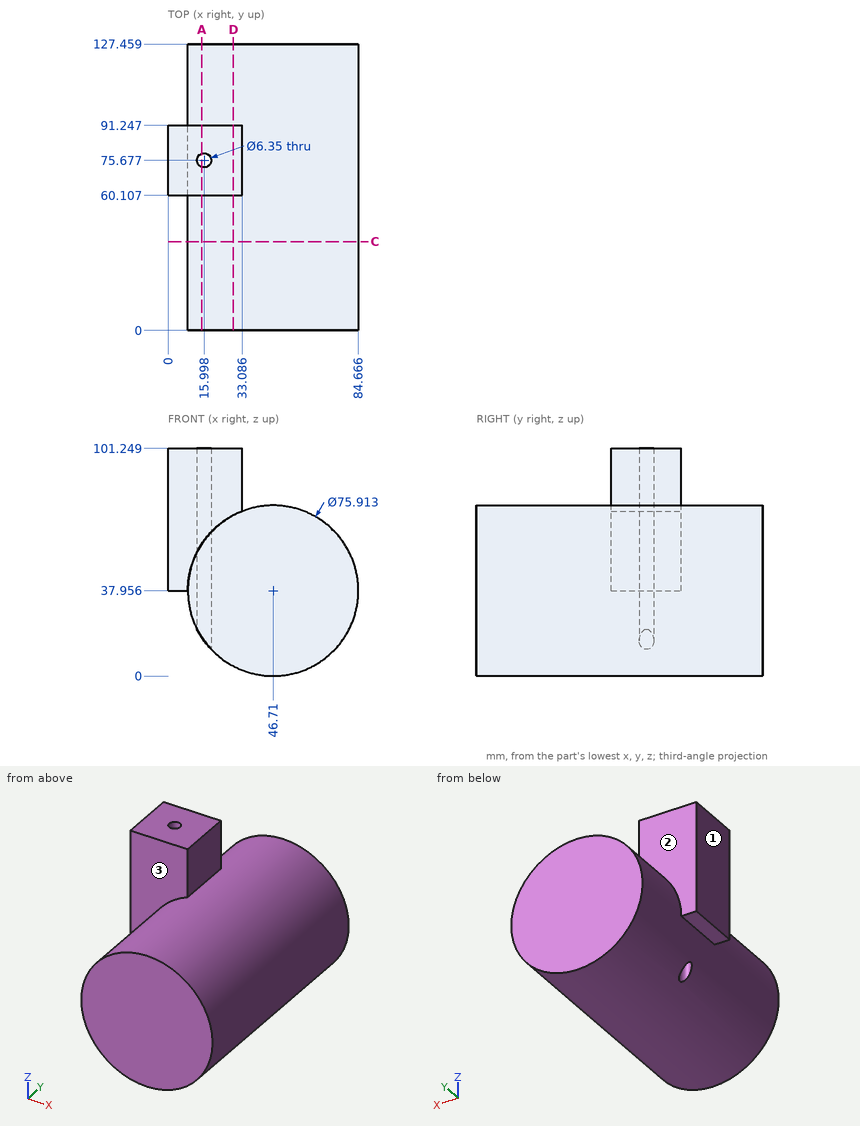
Print and shaded views of the part. All mm, measured from the part's lowest x, y and z. A direction names the side the tool comes from. Coordinates: 2 decimals unless noted, no trailing zeros. Loops run counter-clockwise (first coordinate to the right, second up) from the corner with the lowest first, then second, coordinate; pieces in that order, holes last. Notation, with made-up numbers: (-37.75, 57) -> (-24.75, 57) arc R16 ccw to (-24.75, 61) -> close; hole circle Ø4 at (39, 5). An arc over 180 degrees is marked (long way). Use a Markdown table: item, result. Add a question column.
Item 1: Band-saw the part on A-A on x = 15. Write the cut outline in (y, z) (1 decimal), plus the area to 3 significant figures.
Item 2: Band-saw the part on D-D on x = 29. Write the cut outline in (y, z) (1 decimal).
Item 3: Probe probe 1 along Z at (x, y) = (6, 72); probe 2 along X at (y, z) = (61.5, 82.5); probe 3 along X at (y, z) = (75, 35.5) (1 decimal). List the from-to ranges inside material, lowest first.
Item 4: Which spindle directions (+Z, -Z, +X, -X, +Y, -Y) get a long thin tool onto all of the face, cutting with end or side? Do the marked faces 1, 2 and 3. Say none if no direction does.
Item 5: Band-saw the part on C-C on y = 39.5. Write the cut outline in (x, z).
Item 6: Flat gauge pins, fed straight in: P1, Ø5, axis at x = 24.5, y = 51.5, coming from the -Z side; P2, Ø5, axis at x = 11.5, y = 98.5, coming from the -Z side; P3, Ø16.5, axis at x = 10, z = 68, coming from the -Y side; P4, Ø5.5, axis at x = 16, y = 75.68, coming from the +Z side. Where does each tip first touch, or does it go through?
Geometry says:
| question | item | result |
|---|---|---|
| 1 | outline | (0, 17.1) -> (72.7, 17.1) -> (72.7, 101.2) -> (60.1, 101.2) -> (60.1, 58.8) -> (0, 58.8) -> close; (78.7, 17.1) -> (127.5, 17.1) -> (127.5, 58.8) -> (91.2, 58.8) -> (91.2, 101.2) -> (78.7, 101.2) -> close |
| 1 | area | 6,130 mm² |
| 2 | outline | (0, 4.4) -> (127.5, 4.4) -> (127.5, 71.5) -> (91.2, 71.5) -> (91.2, 101.2) -> (60.1, 101.2) -> (60.1, 71.5) -> (0, 71.5) -> close |
| 3 | probe 1 | 37.96 to 101.25 |
| 3 | probe 2 | 0 to 33.09 |
| 3 | probe 3 | 8.8 to 12.9, 19.1 to 84.6 |
| 4 | face 1 | +Z, -Z, -X, +Y, -Y |
| 4 | face 2 | +Z, -X, +Y |
| 4 | face 3 | +Z, -X, -Y |
| 5 | outline | circle Ø75.91 at (46.71, 37.96) |
| 6 | P1 | z = 5.52 |
| 6 | P2 | z = 18.7 |
| 6 | P3 | y = 60.11 |
| 6 | P4 | through |
